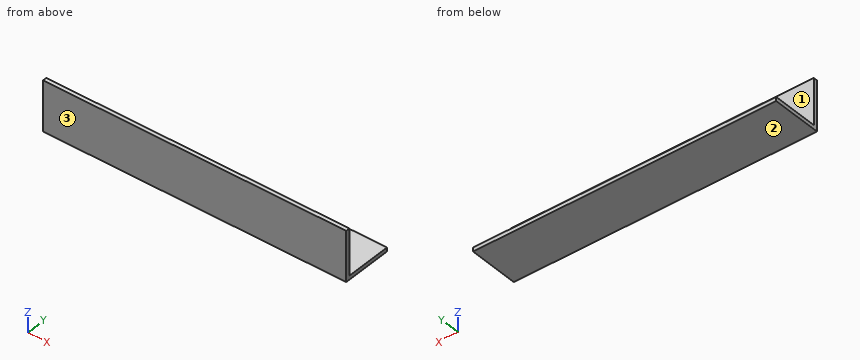
Autodesk Inventor part; units mm, degrees
ref_plane "YZ Plane" through (0, 0, 0) normal (1, 0, 0) x (0, 1, 0)
ref_plane "XZ Plane" through (0, 0, 0) normal (0, 1, 0) x (-1, 0, 0)
ref_plane "XY Plane" through (0, 0, 0) normal (0, 0, 1) x (1, 0, 0)
sketch "Sketch1" plane through (0, 0, 0) normal (0, 0, 1) x (1, 0, 0)
  line L0 (0, 0) -> (230, 0)
  line L1 (230, 0) -> (230, 38)
  line L2 (230, 38) -> (0, 38)
  line L3 (0, 38) -> (0, 0)
  dimension "d0" = 230
  dimension "d1" = 38
extrude "Extrusion1" add sketch "Sketch1" against normal blind 3
sketch "Sketch2" plane through (0, 0, 0) normal (0, 0, 1) x (1, 0, 0)
  line L0 (0, 0) -> (0, 38)
  line L1 (0, 0) -> (230, 0)
  line L2 (230, 0) -> (230, 3)
  line L3 (230, 3) -> (0, 3)
  line L4 (0, 3) -> (0, 0)
  dimension "d4" = 230
  dimension "d5" = 3
extrude "Extrusion2" add sketch "Sketch2" along normal blind 35
properties part number "AluminiumAngle"
Work out the finished part from the listing and answer in its coordinate system (mm). Face numbers are marked on the shaded views. Round coordinates to 2 decimals unless told otherwise and drop trailing zeros. Write each loop counter-clockwise with the first axis right and the second up, starting at its lowest first coordinate (ties: lowest second). Pieces come first, ordered by that corner, then holes. Notation, with made-up numbers: (82, 0.5) - (135, 0.5) arc R36 cw to (135, 36.5) - close; hole circle Ø9 at (-32, 17). An arc over 180 degrees is marked (long way). Return JSON: item names as keys, results as strings. Group by question number.
Q1. Find the intervals of material crossed by L1, parallel to Z at x = 86, y = 8; L2, parallel to Y at x = 146, z = 9, in increasing order.
Q2. The part is cut by section C-C on y = 21. Write down the section's boundary in (x, z), then the cut area to 3 significant figures.
Q3. The part is cut by section B-B on x = 90. Write down the section's boundary in (y, z), then the cut area to 3 significant figures.
Q4. Each of these flat-tipped pins is pushed along its axis until it touches: pin 1 Ø6 at (y, z) = (6.5, 8.5) entering from -X (3 decimals); pin 2 Ø2 at (x, z) = (137.5, 10) entering from +Y; pin 3 Ø12 at (y, z) = (5, 11.5) entering from -X; pin 4 Ø1.5 at (x, y) = (81, 33) entering from +Z. Where does it stop, or does it pass through?
Q5. The mould has two halves that part along Y. Classify the marked faces 1, 2 and 3: released by +Y, released by -Y, zero draft, split by the parting line, or undercut.
Q6. The part is cut by section A-A on z = 9. Write down the section's boundary in (x, y).
Solved:
{
 "1": {"L1": "-3 to 0", "L2": "0 to 3"},
 "2": {"outline": "(0, -3) - (230, -3) - (230, 0) - (0, 0) - close", "area": "690 mm²"},
 "3": {"outline": "(0, -3) - (38, -3) - (38, 0) - (3, 0) - (3, 35) - (0, 35) - close", "area": "219 mm²"},
 "4": {"pin 1": "through", "pin 2": "y = 3", "pin 3": "x = 0", "pin 4": "z = 0"},
 "5": {"face 1": "released by +Y", "face 2": "zero draft", "face 3": "released by -Y"},
 "6": {"outline": "(0, 0) - (230, 0) - (230, 3) - (0, 3) - close"}
}
